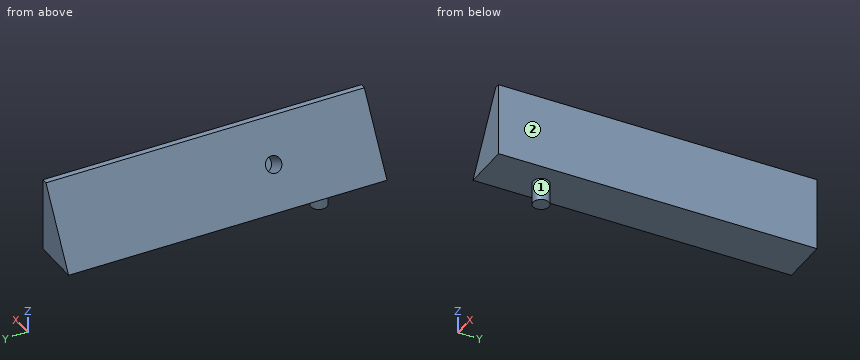
from build123d import *

# Parameters (mm, degrees)
PAD_DEPTH    = 50
SKETCH001_R  = 2.5
PAD001_DEPTH = 7
SKETCH002_R  = 2.5
POCKET_DEPTH = 7


with BuildPart() as part:
    # Sketch → Pad (new body, symmetric)
    with BuildSketch(Plane.XZ):
        Polygon((0, 0), (0, 22.9807621135), (-1.7320508076, 22.9807621135), (-15, 0), align=None)
    extrude(amount=PAD_DEPTH, both=True)

    # Sketch001 (on DatumPlane) → Pad001 (join)
    with BuildSketch(Plane(origin=(0, 0, 0), x_dir=(1, 0, 0), z_dir=(0, 0, -1))):
        with Locations((-7.5, 32.6343382758)):
            Circle(SKETCH001_R)
    extrude(amount=PAD001_DEPTH)

    # Sketch002 (on Face6 of Pad001) → Pocket (cut)
    with BuildSketch(Plane(origin=(-11.25, 0, 6.4951905284), x_dir=(-0.5, 0, -0.8660254038), z_dir=(-0.8660254038, 0, 0.5))):
        with Locations((-5.7679491924, 17.9491805705)):
            Circle(SKETCH002_R)
    extrude(amount=-POCKET_DEPTH, mode=Mode.SUBTRACT)


solid = part.part
Build history of the part. All positions in model axes, mm. Face numbers are marked on the shaded views. A direction names the side the tool comes from. Round coordinates to 2 decimals unless told otherwise and drop trailing zeros. Order: outer loops, then holes, each group sorted by start corner. A loop starts at its lowest first (then second) coordinate and runs counter-clockwise, first axis right, second up. Notation, with made-up numbers: M -17,-18 L 11,-18 A12 ccw 11,-8 Z; hole C 33,-21.75 d10. An arc over 180 degrees is marked long. Use CSV: the item, a comma, the result in double quotes. Start each with the question number.
(1) Drill centre lines: probe 1 along Z at (x, y) = (-1.25, -34.5); probe 2 along X at (y, z) = (-6, 15); probe 3 along Z at (x, y) = (-5.25, -42.5). Where is each one in solid material? Low to high.
(2) Cut at A-A on y = -5.5. List the corners of the cut face in (x, z).
(3) Flat gauge pins, fed straight in: P1, Ø2, axis at y = 0, z = 8, coming from the -X side; P2, Ø8, axis at x = -10, y = -38.5, coming from the -Z side; P3, Ø1.5, axis at x = -9.5, y = -9, coming from the -Z side; P4, Ø2, axis at y = -10, z = -1.5, coming from the +X side. Where does each tip first touch, or does it go through?
(4) Tool access for the marked faces 1 and 2: list every direction of +Z, -Z, +X, -X, +Y, -Y with a clear straight run to the whole face (end or side of a thin tool).
(5) Cut at B-B on x = -11.25. List the corners of the cut face in (y, z).
Findings:
1,probe 1,"z = 0 to 22.98"
1,probe 2,"x = -6.34 to 0"
1,probe 3,"z = 0 to 16.89"
2,outline,"M -15,0 L 0,0 L 0,22.98 L -1.73,22.98 Z"
3,P1,"stops at x = -10.96"
3,P2,"stops at z = -7"
3,P3,"stops at z = 0"
3,P4,"passes through"
4,face 1,"-Z"
4,face 2,"+Z, -Z, +X, +Y, -Y"
5,outline,"M -50,0 L 50,0 L 50,6.5 L -50,6.5 Z"
